from build123d import *

# Parameters (mm, degrees)
SKETCH_1_W           = 82
SKETCH_1_H           = 58
EXTRUDE_1_DEPTH      = 42
SKETCH_2_OUTSIDE_W   = 105.774
SKETCH_2_OUTSIDE_H   = 81.774
SKETCH_2_OUTSIDE_W_2 = 77
SKETCH_2_OUTSIDE_H_2 = 54
CUT_EXTRUDE_1_DEPTH  = 40
SKETCH_3_R           = 2.051183763
SKETCH_3_R_2         = 1.551183763
SKETCH_3_W           = 76.662993142
SKETCH_3_H           = 44.9978438
SKETCH_3_W_2         = 75.662993142
SKETCH_3_H_2         = 43.9978438
CUT_EXTRUDE_2_DEPTH  = 2
SKETCH_5_W           = 56.22095986
SKETCH_5_H           = 0.839970392
CUT_EXTRUDE_3_DEPTH  = 2


with BuildPart() as part:
    # 草图1 → 凸台-拉伸1 (new body)
    with BuildSketch(Plane.XY):
        Rectangle(SKETCH_1_W, SKETCH_1_H)
    extrude(amount=-EXTRUDE_1_DEPTH)

    # 草图2 outside → 切除-拉伸1 (cut)
    with BuildSketch(Plane(origin=(0, 0, -42), x_dir=(-1, 0, 0), z_dir=(0, 0, -1))):
        Rectangle(SKETCH_2_OUTSIDE_W, SKETCH_2_OUTSIDE_H)
        Rectangle(SKETCH_2_OUTSIDE_W_2, SKETCH_2_OUTSIDE_H_2, mode=Mode.SUBTRACT)
    extrude(amount=-CUT_EXTRUDE_1_DEPTH, mode=Mode.SUBTRACT)

    # 草图3 → 切除-拉伸2 (cut)
    # profile 1 of 2: a face of its own
    with BuildSketch(Plane.XY):
        with Locations((-37.049506719, -24.324267733)):
            Circle(SKETCH_3_R)
        with Locations((-37.049506719, -24.324267733)):
            Circle(SKETCH_3_R_2, mode=Mode.SUBTRACT)
    # profile 2 of 2: a face of its own
    with BuildSketch(Plane.XY):
        with Locations((0, 3.943608501)):
            Rectangle(SKETCH_3_W, SKETCH_3_H)
        with Locations((0, 3.943608501)):
            Rectangle(SKETCH_3_W_2, SKETCH_3_H_2, mode=Mode.SUBTRACT)
    extrude(amount=-CUT_EXTRUDE_2_DEPTH, mode=Mode.SUBTRACT)

    # 草图5 → 切除-拉伸3 (cut)
    # profile 1 of 2: a face of its own
    with BuildSketch(Plane.XY):
        with Locations((0, -18.975298595)):
            Rectangle(SKETCH_5_W, SKETCH_5_H)
    # profile 2 of 2: a face of its own
    with BuildSketch(Plane.XY):
        with BuildLine():
            Line((22.181492686, -2.55676808), (-22.181492686, -2.55676808))
            Line((-22.181492686, -2.55676808), (-22.181492686, 5.66529789))
            add(Edge.make_bspline(
                [(-22.181492686, 5.66529789), (-21.613171528, 6.595019079), (-20.324411635, 8.382514153), (-17.243691235, 11.385794253), (-12.622221003, 14.216373785), (-7.423291418, 15.868320573), (-3.158321809, 16.537625375), (-1.057172799, 16.660943148), (0, 16.672230501)],
                knots=[-0.005481994, -0.005481994, -0.005481994, -0.005481994, 0.120230411, 0.245942817, 0.497367628, 0.748792439, 0.874504845, 1.00021725, 1.00021725, 1.00021725, 1.00021725], degree=3))
            add(Edge.make_bspline(
                [(0, 16.672230501), (1.057172799, 16.660943148), (3.158321809, 16.537625375), (7.423291418, 15.868320573), (12.622221003, 14.216373785), (17.243691235, 11.385794253), (20.324411635, 8.382514153), (21.613171528, 6.595019079), (22.181492686, 5.66529789)],
                knots=[-0.005481994, -0.005481994, -0.005481994, -0.005481994, 0.120230411, 0.245942817, 0.497367628, 0.748792439, 0.874504845, 1.00021725, 1.00021725, 1.00021725, 1.00021725], degree=3))
            Line((22.181492686, 5.66529789), (22.181492686, -2.55676808))
        make_face()
        with BuildLine():
            Line((21.693569538, -2.05676808), (-21.693569538, -2.05676808))
            Line((-21.693569538, -2.05676808), (-21.693569538, 3.576865713))
            add(Edge.make_bspline(
                [(-21.693569538, 3.576865713), (-17.048272024, 10.504797519), (-7.443342261, 11.136498571), (0, 11.122264619)],
                knots=[0, 0, 0, 0, 1, 1, 1, 1], degree=3))
            add(Edge.make_bspline(
                [(21.693569538, 3.576865713), (17.048272024, 10.504797519), (7.443342261, 11.136498571), (0, 11.122264619)],
                knots=[0, 0, 0, 0, 1, 1, 1, 1], degree=3))
            Line((21.693569538, 3.576865713), (21.693569538, -2.05676808))
        make_face(mode=Mode.SUBTRACT)
    extrude(amount=-CUT_EXTRUDE_3_DEPTH, mode=Mode.SUBTRACT)


solid = part.part
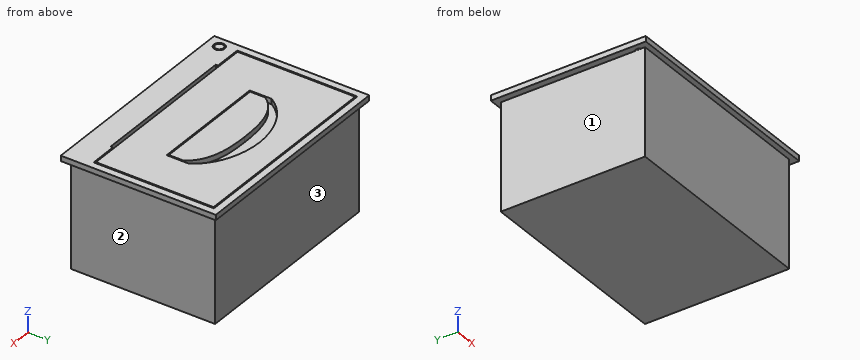
Can you work these out from the model? Positions are in its coordinate system, mm. Face numbers are marked on the shaded views. A direction names the side the tool comes from. Coordinates: 2 decimals unless noted, no trailing zeros. Write each loop counter-clockwise with the first axis right and the second up, starting at its lowest first coordinate (ties: lowest second). Pieces come first, ordered by that corner, then holes. Notation, with made-up numbers: (62.25, 35) -> (88.25, 35) arc R33 ccw to (88.25, 68) -> close; hole circle Ø10 at (68.5, 34). An arc over 180 degrees is marked (long way). Write each question's results on one line, items separated by ' | '. Start each with the question number.
Item 1: I'm going to push flat-ended pins straight in: P1, Ø12, axis at x = 17.5, z = -23, coming from the -Y side; P2, Ø5, axis at y = -13, z = -14.5, coming from the +X side; P3, Ø5, axis at x = -19, z = -25, coming from the +Y side. Where does each tip first touch, or does it pass through?
Item 2: If we section it at C-C, the plane z = -18.5: Write out the boundary of the cut face in (x, y).
Item 3: If we section it at B-B, the plane y = -13.5: Write out the boundary of the cut face in (x, z), and give its area (3 significant figures).
Item 4: If we section it at A-A, the plane x = 24: Write out the boundary of the cut face in (y, z), and give its area (3 significant figures).
Item 5: On a 3-axis mill with a long thin cutter (end or side, diameter ignored), from which of +Z, -Z, +X, -X, +Y, -Y can I reach the whole of each face in a straight line? I mean the marked faces 1, 2 and 3. Say none if no direction works.
Item 6: Please list where these lines run through material, in increasing order: probe 1 along Y at (x, z) = (-1, -22); probe 2 along X at (y, z) = (6, -25.5).
Item 7: If we section it at D-D, the plane y = 1.5: Write out the boundary of the cut face in (x, z), and give its area (3 significant figures).
Answer block:
1) P1: y = -27 | P2: x = 38.5 | P3: y = 27
2) outline: (-38.5, -27) -> (38.5, -27) -> (38.5, 27) -> (-38.5, 27) -> close
3) outline: (-41, -2) -> (-38.5, -2) -> (-38.5, -42) -> (38.5, -42) -> (38.5, -2) -> (41, -2) -> (41, 0) -> (38.33, 0) -> (38.33, -2) -> (37.83, -2) -> (37.83, 0) -> (-37.83, 0) -> (-37.83, -2) -> (-38.33, -2) -> (-38.33, 0) -> (-41, 0) -> close | area: 3,240 mm²
4) outline: (-29, -2) -> (-27, -2) -> (-27, -42) -> (27, -42) -> (27, -2) -> (29, -2) -> (29, 0) -> (26.44, 0) -> (26.44, -2) -> (25.94, -2) -> (25.94, 0) -> (-18.06, 0) -> (-18.06, -2) -> (-19.4, -2) -> (-19.4, 0) -> (-29, 0) -> close | area: 2,270 mm²
5) face 1: -Z, -X, +Y, -Y | face 2: -Z, +X, +Y, -Y | face 3: -Z, +X, -X, +Y
6) probe 1: -27 to 27 | probe 2: -38.5 to 38.5
7) outline: (-41, -2) -> (-38.5, -2) -> (-38.5, -42) -> (38.5, -42) -> (38.5, -2) -> (41, -2) -> (41, 0) -> (38.33, 0) -> (38.33, -2) -> (37.83, -2) -> (37.83, 0) -> (22.18, 0) -> (22.18, -2) -> (21.69, -2) -> (21.69, 0) -> (-21.69, 0) -> (-21.69, -2) -> (-22.18, -2) -> (-22.18, 0) -> (-37.83, 0) -> (-37.83, -2) -> (-38.33, -2) -> (-38.33, 0) -> (-41, 0) -> close | area: 3,240 mm²
